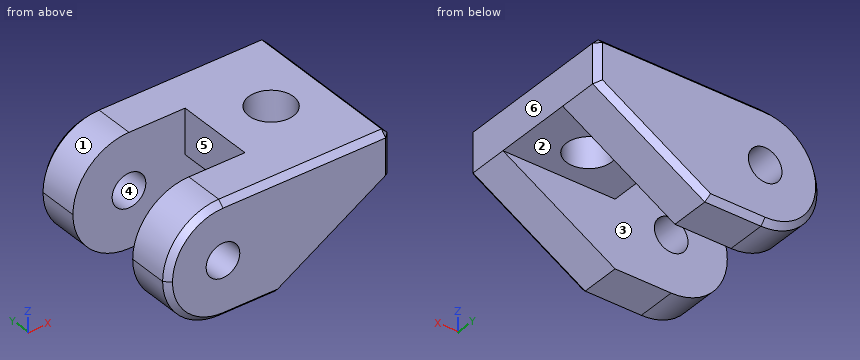
```python
from build123d import *

# Parameters (mm, degrees)
EXTRUDE_1_DEPTH     = 15
SKETCH_2_W          = 10
SKETCH_2_H          = 7
CUT_EXTRUDE_1_DEPTH = 27.925824036
SKETCH_3_W          = 6
SKETCH_3_H          = 7
CUT_EXTRUDE_2_DEPTH = 21.615528128
SKETCH_4_R          = 2
CUT_EXTRUDE_3_DEPTH = 26.709920264
FILLET_1_R          = 5
SKETCH_5_R          = 1.5
CUT_EXTRUDE_4_DEPTH = 27.925824036
CHAMFER_1_SIZE      = 0.5


with BuildPart() as part:
    # ｽｹｯﾁ1 → ﾎﾞｽ - 押し出し1 (new body)
    with BuildSketch(Plane(origin=(0, 0, 0), x_dir=(1, 0, 0), z_dir=(0, 1, 0))):
        Polygon((0, 0), (20, 0), (20, 4), (10, 10), (0, 10), align=None)
    extrude(amount=EXTRUDE_1_DEPTH)

    # ｽｹｯﾁ2 → ｶｯﾄ - 押し出し1 (cut, through all)
    with BuildSketch(Plane(origin=(0, 0, -10), x_dir=(-1, 0, 0), z_dir=(0, 0, -1))):
        with Locations((-5, 7.5)):
            Rectangle(SKETCH_2_W, SKETCH_2_H)
    extrude(amount=-CUT_EXTRUDE_1_DEPTH, mode=Mode.SUBTRACT)

    # ｽｹｯﾁ3 → ｶｯﾄ - 押し出し2 (cut, through all)
    with BuildSketch(Plane.ZY.offset(-10)):
        with Locations((-7, 7.5)):
            Rectangle(SKETCH_3_W, SKETCH_3_H)
    extrude(amount=-CUT_EXTRUDE_2_DEPTH, mode=Mode.SUBTRACT)

    # ｽｹｯﾁ4 → ｶｯﾄ - 押し出し3 (cut, through all)
    with BuildSketch(Plane(origin=(0, 0, -4), x_dir=(-1, 0, 0), z_dir=(0, 0, -1))):
        with Locations((-15, 7.5)):
            Circle(SKETCH_4_R)
    extrude(amount=-CUT_EXTRUDE_3_DEPTH, mode=Mode.SUBTRACT)

    # ﾌｨﾚｯﾄ1
    fillet_1_edges = [part.edges().sort_by_distance(p)[0] for p in [
        (0, 2, 0),
        (0, 2, -10),
        (0, 13, 0),
        (0, 13, -10),
    ]]
    fillet(fillet_1_edges, radius=FILLET_1_R - 0.0001)  # a hair under: the kernel refuses the full size

    # ｽｹｯﾁ5 → ｶｯﾄ - 押し出し4 (cut, through all)
    with BuildSketch(Plane.XZ):
        with Locations(Location((5, -5, 0), (0, 0, 270))):
            Circle(SKETCH_5_R)
    extrude(amount=-CUT_EXTRUDE_4_DEPTH, mode=Mode.SUBTRACT)

    # 面取り1
    chamfer_1_edges = [part.edges().sort_by_distance(p)[0] for p in [
        (20, 15, -2),
        (15, 15, -7),
        (7.49995, 15, -10),
        (7.49995, 0, -10),
        (12.49995, 0, 0),
        (12.49995, 15, 0),
        (15, 0, -7),
        (1.464436805, 0, -8.535563195),
        (1.464436805, 0, -1.464436805),
        (20, 0, -2),
        (1.464436805, 15, -8.535563195),
        (1.464436805, 15, -1.464436805),
        (20, 7.5, 0),
    ]]
    chamfer(chamfer_1_edges, length=CHAMFER_1_SIZE)


solid = part.part
```
Source: CAD feature listing. Evaluate the final solid. Frame: model axes, mm. Face numbers are marked on the shaded views. A direction names the side the tool comes from. Coordinates: 2 decimals unless noted, no trailing zeros. Loops run counter-clockwise (first coordinate to the right, second up) from the corner with the lowest first, then second, coordinate; pieces in that order, holes last. Notation, with made-up numbers: (53, 12.5) -> (99, 12.5) arc R32 ccw to (99, 46.5) -> close; hole circle Ø5 at (73.5, 31.5). An arc over 180 degrees is marked (long way). One line per item, written item: value. Start each with the question number.
Q1. Section query C-C, the plane y = 6.5. Return the cut outline in (x, z), and give its area (3 significant figures).
Q2. Contact query for flat-ended pins moving along their axis: P1, Ø3.5, axis at x = 5, z = -5, coming from the +Y side; P2, Ø1.5, axis at x = 17.5, y = 3, coming from the -Z side; P3, Ø4.5, axis at y = 8.5, z = -3, coming from the -X side. Output: stop coordinate, or through.
Q3. Mould query, pull axis X, two halves, no side actions, for the marked faces 4, 5 and 6. Classes: pulls with the +X half, pulls with the -X half, needs draft (parallel to the pull), parting line crosses it, or undercut.
Q4. Section query B-B, the plane x = 16.5. Return the cut outline in (y, z).
Q5. Set-up query: the marked faces 1, 2 and 3. Return all of +Z, -Z, +X, -X, +Y, -Y with unobstructed straight access to the full face (end or side cutting, diameter ignored); none if empty.
Q6. Section query D-D, the plane z = -4.5. Give the number of separate pieces and of enclosed holes in the cut face, and give its area (3 significant figures).
Q7. Line query: line 1 along Y through (x, z) = (8.5, -6.25); line 2 along Z through (x, y) = (14, 10.25); line 3 along X through (y, z) = (14.2, -5). Output: solid intervals per line, ascending.
Results:
1. outline: (10, -4) -> (13.27, -4) -> (13.27, 0) -> (10, 0) -> close; (16.73, -4) -> (20, -4) -> (20, -0.5) -> (19.5, 0) -> (16.73, 0) -> close
1. area: 26.0 mm^2
2. P1: y = 15
2. P2: z = -5.95
2. P3: x = 10
3. face 4: undercut
3. face 5: pulls with the -X half
3. face 6: pulls with the +X half
4. outline: (0, -5.52) -> (0.5, -6.1) -> (4, -6.1) -> (4, -4) -> (6.18, -4) -> (6.18, 0) -> (0.5, 0) -> (0, -0.5) -> close; (8.82, -4) -> (11, -4) -> (11, -6.1) -> (14.5, -6.1) -> (15, -5.52) -> (15, -0.5) -> (14.5, 0) -> (8.82, 0) -> close
5. face 1: +Z, -X, +Y, -Y
5. face 2: -Z, +X, -X
5. face 3: -Z, -X
6. separate pieces: 4
6. enclosed holes: 0
6. area: 130 mm^2
7. line 1: 0 to 4, 11 to 15
7. line 2: -4 to 0
7. line 3: 0 to 3.5, 6.5 to 18.33
